The listing builds one solid part. Answer for the finished solid, in the listing's coordinates (mm). Give positions to 0.01 mm unless a question says otherwise; leave off trailing zeros. Write each loop counter-clockwise with the first axis right and the second up, starting at its lowest first coordinate (ties: lowest second). Pieces come first, ordered by that corner, then holes. Notation, with made-up numbers: (69, 49.25) -> (101, 49.25) arc R33 ccw to (101, 87.25) -> close; hole circle Ø3 at (24, -9). An arc over 180 degrees is marked (long way). Put each result on its own line as item: value. Start each with the question number.
1) A cutting plane is placed at B-B (x = 4). Write down the section's boundary in (y, z), then the cut area to 3 significant figures.
2) A cutting plane is placed at A-A (z = 5.5). Give the number of separate pieces and of enclosed holes in the cut face, then the cut area to 3 significant figures.
3) Find the intervals of material crossed by line 1 along Z through (x, y) = (0.5, 8.1), in increasing order. Write a range as from..to.
4) A flat-ended cylindrical pin translates along its axis: pin 1 Ø5 at (x, z) = (-6, 2.5) entering from +Y. Find the tip coordinate at first contact, or state that the pin passes through.
from build123d import *

# Parameters (mm, degrees)
SKETCH006_W            = 30.48
SKETCH006_H            = 8.74
PAD014_DEPTH           = 0.3
SKETCH007_W            = 1.94
SKETCH007_H            = 12.4
POCKET002_DEPTH        = 0.301
POCKET002_DEPTH_BACK   = 0.301
LINEARPATTERN002_COUNT = 12
LINEARPATTERN002_PITCH = 2.770909
LINEARPATTERN003_COUNT = 12
LINEARPATTERN003_PITCH = 2.770909


with BuildPart() as part:
    # Sketch006 → Pad014 (new body, symmetric)
    with BuildSketch(Plane.XZ):
        with Locations((0, 4.37)):
            Rectangle(SKETCH006_W, SKETCH006_H)
    extrude(amount=PAD014_DEPTH, both=True)

    # Sketch007 → Pocket002 (cut, two sides)
    with BuildSketch(Plane.XZ) as pocket002_sk:
        with Locations((-1.27, 8.44)):
            Rectangle(SKETCH007_W, SKETCH007_H)
        with Locations((1.27, 8.44)):
            Rectangle(SKETCH007_W, SKETCH007_H)
    pocket002 = extrude(amount=-POCKET002_DEPTH, mode=Mode.SUBTRACT) + extrude(pocket002_sk.sketch, amount=POCKET002_DEPTH_BACK, mode=Mode.SUBTRACT)

    # LinearPattern002: Pocket002 ×12
    with Locations(*[(i * LINEARPATTERN002_PITCH, 0, 0) for i in range(1, LINEARPATTERN002_COUNT)]):
        add(pocket002, mode=Mode.SUBTRACT)

    # LinearPattern003: Pocket002 ×12
    with Locations(*[(-i * LINEARPATTERN003_PITCH, 0, 0) for i in range(1, LINEARPATTERN003_COUNT)]):
        add(pocket002, mode=Mode.SUBTRACT)


with BuildPart() as part_1:
    # Body022 placement: moved
    add(part.part.moved(Location((0, -8, 0))))


with BuildPart() as part_2:
    # Body025 placement: moved
    add(part_1.part.moved(Location((0, 16, 0))))


solid = part_2.part
Reply:
1. outline: (7.7, 0) -> (8.3, 0) -> (8.3, 2.24) -> (7.7, 2.24) -> close
1. area: 1.34 mm2
2. separate pieces: 11
2. enclosed holes: 0
2. area: 3.96 mm2
3. line 1: z = 0..2.24
4. pin 1: stops at y = 8.3
